from build123d import *

# Parameters (mm, degrees)
BOSS_EXTRUDE1_DEPTH = 36
SKETCH1_3_W         = 48
SKETCH1_3_H         = 12
BOSS_EXTRUDE2_DEPTH = 48
SKETCH1_4_W         = 48
SKETCH1_4_H         = 16
BOSS_EXTRUDE3_DEPTH = 24
FILLET1_R           = 0.5


with BuildPart() as part:
    # Sketch1 → Boss-Extrude1 (new body)
    with BuildSketch(Plane(origin=(0, 0, 0), x_dir=(0, 0, -1), z_dir=(1, 0, 0))):
        Polygon((-36, 0), (-36, -12), (36, -12), (36, 12), (12, 12), (12, 0), align=None)
    extrude(amount=BOSS_EXTRUDE1_DEPTH)

    # Sketch1<3> → Boss-Extrude2 (add)
    with BuildSketch(Plane(origin=(0, 0, 0), x_dir=(0, 0, -1), z_dir=(1, 0, 0))):
        with Locations((-12, 6)):
            Rectangle(SKETCH1_3_W, SKETCH1_3_H)
    extrude(amount=BOSS_EXTRUDE2_DEPTH)

    # Sketch1<4> → Boss-Extrude3 (add)
    with BuildSketch(Plane(origin=(0, 0, 0), x_dir=(0, 0, -1), z_dir=(1, 0, 0))):
        with Locations((-12, 20)):
            Rectangle(SKETCH1_4_W, SKETCH1_4_H)
    extrude(amount=BOSS_EXTRUDE3_DEPTH)

    # Fillet1
    fillet1_edges = [part.edges().sort_by_distance(p)[0] for p in [
        (36, 0, 12),
        (18, 12, -36),
        (18, -12, -36),
        (18, -12, 36),
        (36, -6, 36),
        (36, -12, 0),
        (42, 0, 36),
        (48, 0, 12),
        (42, 0, -12),
        (48, 6, -12),
        (48, 12, 12),
        (42, 12, -12),
        (48, 6, 36),
        (36, 12, 36),
        (36, 0, -36),
        (36, 12, -24),
        (0, 12, -24),
        (0, 20, -12),
        (12, 12, -12),
        (24, 28, 12),
        (12, 28, -12),
        (24, 20, 36),
        (12, 28, 36),
        (24, 12, 12),
        (24, 20, -12),
        (0, 28, 12),
        (36, 6, -12),
        (0, 0, -36),
        (0, -12, 0),
        (0, 8, 36),
    ]]
    fillet(fillet1_edges, radius=FILLET1_R)


solid = part.part
Source: CAD feature listing. Evaluate the final solid. Frame: model axes, mm. A direction names the side the tool comes from. Round coordinates to 2 decimals unless told otherwise and drop trailing zeros. Loops run counter-clockwise (first coordinate to the right, second up) from the corner with the lowest first, then second, coordinate; pieces in that order, holes last.
Q1. First-contact query: P1, Ø5.5, axis at x = 44, z = 17, coming from the -Y side; P2, Ø1.5, axis at y = 6, z = -17, coming from the +X side; P3, Ø6, axis at x = 37.5, z = -26.5, coming from the +Y side. Flat tips, straight axial feed; report the tip coordinate or a pass-through.
Q2. Section D-D, the plane y = 2.5. Return loops of the section in (x, z), plus the area to 3 significant figures.
Q3. Section C-C, the plane x = 4. Return loops of the section in (y, z), plus the area to 3 significant figures.
Q4. Section A-A, the plane y = -4. Return loops of the section in (x, z).
Q5. Access query for faces 1 (the face through (42, 6, -12)), 2 (the face through (12, 20, -12)), 3 (the face through (24, 20, 12)), 4 (the face through (29, 12, -7)). Directions: +Z, -Z, +X, -X, +Y, -Y. A direction counts if a zero-diameter tool reaches every point of the face in a straight line with its end or side. Return the directions, or none.
Q6. Section B-B, the plane z = -20.5. Return loops of the section in (x, y), plus the area to 3 significant figures.
Q7. Ray query, line 1 (X direction, y = 9, z = -19.5); line 2 (Z direction, x = 11, y = 23); line 3 (Y direction, x = 43, z = -10.5). Return the intervals inside material, ascending.
Solutions:
1. P1: stops at y = 0
1. P2: stops at x = 36
1. P3: stops at y = 12
2. outline: (0, -35.5) arc R0.5 ccw to (0.5, -36) - (35.5, -36) arc R0.5 ccw to (36, -35.5) - (36, -12.5) arc R0.5 cw to (36.5, -12) - (47.5, -12) arc R0.5 ccw to (48, -11.5) - (48, 35.5) arc R0.5 ccw to (47.5, 36) - (0.5, 36) arc R0.5 ccw to (0, 35.5) - close
2. area: 3,170 mm2
3. outline: (-12, -35.5) arc R0.5 ccw to (-11.5, -36) - (11.5, -36) arc R0.5 ccw to (12, -35.5) - (12, -12.5) arc R0.5 cw to (12.5, -12) - (27.5, -12) arc R0.5 ccw to (28, -11.5) - (28, 35.5) arc R0.5 ccw to (27.5, 36) - (-11.5, 36) arc R0.5 ccw to (-12, 35.5) - close
3. area: 2,500 mm2
4. outline: (0, -35.5) arc R0.5 ccw to (0.5, -36) - (35.5, -36) arc R0.5 ccw to (36, -35.5) - (36, 35.5) arc R0.5 ccw to (35.5, 36) - (0.5, 36) arc R0.5 ccw to (0, 35.5) - close
5. face 1: -Z, +X, +Y, -Y
5. face 2: -Z, +X, -X, +Y
5. face 3: +Z, -Z, +X, +Y
5. face 4: -Z, +X, +Y
6. outline: (0, -11.5) arc R0.5 ccw to (0.5, -12) - (35.5, -12) arc R0.5 ccw to (36, -11.5) - (36, 11.5) arc R0.5 ccw to (35.5, 12) - (0.5, 12) arc R0.5 ccw to (0, 11.5) - close
6. area: 864 mm2
7. line 1: x = 0 to 36
7. line 2: z = -12 to 36
7. line 3: y = 0 to 12
